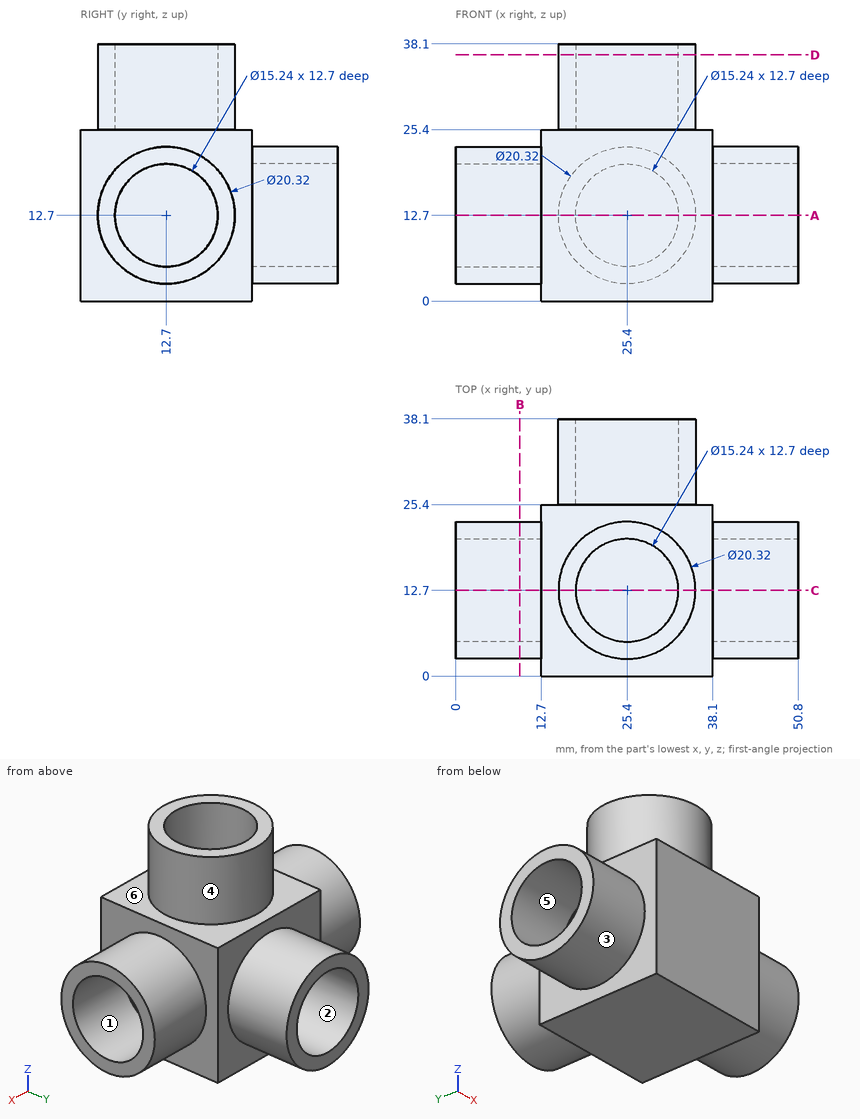
Job drawing, mm, ordinate dimensions from the low corner. One solid piece. A direction names the side the tool comes from. Round coordinates to 2 decimals unless told otherwise and drop trailing zeros. Loops run counter-clockwise (first coordinate to the right, second up) from the corner with the lowest first, then second, coordinate; pieces in that order, holes last. Notation, with made-up numbers: M -18,60.25 L -3,60.25 A16 cw -3,85.25 Z; hole C 71.25,44.25 d8. An arc over 180 degrees is marked long. One line per question, with ' | ' between items. Start each with the question number.
Item 1: Pin check, flat tips, straight feed: pin 1 Ø1 at (x, y) = (30, 27.5) entering from -Z; pin 2 Ø7.5 at (x, y) = (23.5, 12.5) entering from +Z; pin 3 Ø10 at (y, z) = (30.5, 11) entering from -X. Stop position of each tip, or through.
Item 2: Wall check: line 1 (Z direction, x = 25, y = 31); line 2 (Y direction, x = 25.4, z = 33); line 3 (Y direction, x = 23, z = 29). Give the ranges that are in metal, low to high.
Item 3: Cut at B-B, the plane x = 9.5. Write the cut outline in (y, z).
Item 4: Which spindle directions (+Z, -Z, +X, -X, +Y, -Y) get a long thin tool onto all of the face, cutting with end or side? Do the marked faces 1, 2 and 3. Say none if no direction does.
Item 5: Cut at D-D, the plane z = 36.5. Write the cut outline in (x, y).
Item 6: Two-plate mould, pull along Z, no slides. Class the marked faces 4, 5 and 6: pulls with the +Z half, pulls with the -Z half, needs draft (parallel to the pull), parting line crosses it, or undercut.
Item 7: Cut at A-A, the plane z = 12.7. Write the cut outline in (x, y).
Responses:
1) pin 1: stops at z = 3.4 | pin 2: stops at z = 25.4 | pin 3: stops at x = 15.24
2) line 1: z = 2.55 to 5.09, 20.31 to 22.85 | line 2: y = 2.54 to 5.08, 20.32 to 22.86 | line 3: y = 2.83 to 5.47, 19.93 to 22.57
3) outline: C 12.7,12.7 d20.32; hole C 12.7,12.7 d15.24
4) face 1: +X | face 2: +Y | face 3: -X
5) outline: C 25.4,12.7 d20.32; hole C 25.4,12.7 d15.24
6) face 4: needs draft | face 5: undercut | face 6: pulls with the +Z half
7) outline: M 0,2.54 L 12.7,2.54 L 12.7,0 L 38.1,0 L 38.1,2.54 L 50.8,2.54 L 50.8,5.08 L 38.1,5.08 L 38.1,20.32 L 50.8,20.32 L 50.8,22.86 L 38.1,22.86 L 38.1,25.4 L 35.56,25.4 L 35.56,38.1 L 33.02,38.1 L 33.02,25.4 L 17.78,25.4 L 17.78,38.1 L 15.24,38.1 L 15.24,25.4 L 12.7,25.4 L 12.7,22.86 L 0,22.86 L 0,20.32 L 12.7,20.32 L 12.7,5.08 L 0,5.08 Z
